Can you work these out from the drawing? Everything is in mm from the part's minimum corner. A direction names the side the tool comes from. Give positions to 0.01 mm unless a question says otherwise; leave off trailing zeros. Order: outer loops, then holes, each group sorted by start corner. A loop starts at its lowest first (then second) coordinate and runs counter-clockwise, first axis right, second up. Notation, with made-up numbers: (66.5, 39.5) - (125.5, 39.5) arc R25 ccw to (125.5, 78.5) - close; hole circle Ø9 at (68.5, -2). An arc over 180 degrees is marked (long way). One line per question, with ' | ' between items.
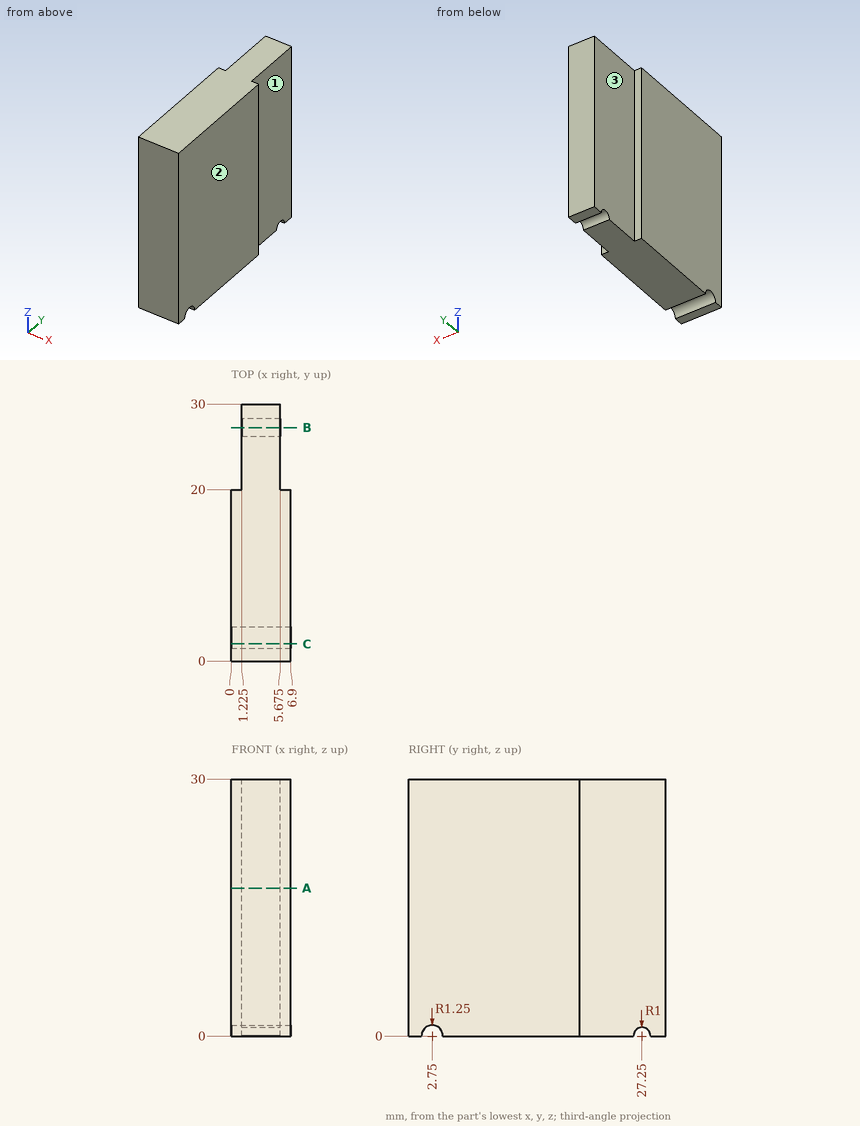
1) I want a section at C-C (y = 2). List the corners of the cut face in (x, z) for me, plus the area to 3 significant figures.
Model answer:
outline: (0, 1) - (6.9, 1) - (6.9, 30) - (0, 30) - close | area: 200 mm2
2) Please list where these lines run through material, in increasing order: L1, parallel to X at y = 27.25, z = 6.75 (3 decimals); L2, parallel to Y at x = 6.75, z = 1.75; L3, parallel to Z at x = 2.25, y = 26.5.
Model answer:
L1: x = 1.225 to 5.675 | L2: y = 0 to 20 | L3: z = 0.66 to 30
3) I want a section at B-B (y = 27.25). List the corners of the cut face in (x, z) for me (3 decimals), plus the area to 3 significant figures.
Model answer:
outline: (1.225, 1) - (5.675, 1) - (5.675, 30) - (1.225, 30) - close | area: 129 mm2
4) I want a section at A-A (z = 17.25). List the corners of the cut face in (x, y) for me (3 decimals).
Model answer:
outline: (0, 0) - (6.9, 0) - (6.9, 20) - (5.675, 20) - (5.675, 30) - (1.225, 30) - (1.225, 20) - (0, 20) - close
5) On a 3-axis mill with a long thin cutter (end or side, diameter ignored), from which of +Z, -Z, +X, -X, +Y, -Y can I reach the whole of each face in a straight line? I mean the marked faces 1, 2 and 3. Say none if no direction works.
Model answer:
face 1: +Z, -Z, +X, +Y | face 2: +Z, -Z, +X, +Y, -Y | face 3: +Z, -Z, -X, +Y
6) I'm going to push flat-ended pins straight in: P1, Ø1.5, axis at y = 21, z = 23.5, coming from the +X side (3 decimals); P2, Ø11, axis at y = 25, z = 14.5, coming from the +X side; P3, Ø3, axis at y = 26.5, z = 16.5, coming from the -X side (3 decimals). Where does each tip first touch, or does it pass through?
Model answer:
P1: stops at x = 5.675 | P2: stops at x = 6.9 | P3: stops at x = 1.225
